from build123d import *

# Parameters (mm, degrees)
SKETCH_W            = 101
SKETCH_H            = 96
PAD_DEPTH           = 23
SKETCH001_W         = 97
SKETCH001_H         = 92
POCKET_DEPTH        = 21
SKETCH002_R         = 6
PAD001_DEPTH        = 5.6
SKETCH003_R         = 1.6
POCKET001_DEPTH     = 7
SKETCH004_R         = 1.6
POCKET002_DEPTH     = 5
SKETCH005_W         = 79
SKETCH005_H         = 52
POCKET003_DEPTH     = 23.001
SKETCH006_R         = 3
PAD002_DEPTH        = 6
POCKET004_DEPTH     = 2.001
LINEARPATTERN_COUNT = 4
LINEARPATTERN_PITCH = 3.333333
SKETCH008_R         = 4
POCKET005_DEPTH     = 2.001
POCKET006_DEPTH     = 2.001
SKETCH010_R         = 3
POCKET007_DEPTH     = 0.5
POCKET008_DEPTH     = 0.5
SKETCH012_W         = 26.5
SKETCH012_H         = 3.3
POCKET009_DEPTH     = 3
CHAMFER_SIZE        = 1.5
FILLET_R            = 1.5
CHAMFER001_SIZE     = 0.5
CHAMFER002_SIZE     = 0.49
SKETCH013_R         = 3.1
POCKET010_DEPTH     = 2.6
CHAMFER003_SIZE     = 1.3


with BuildPart() as part:
    # Sketch → Pad (new body)
    with BuildSketch(Plane.XZ):
        with Locations((50.5, 48)):
            Rectangle(SKETCH_W, SKETCH_H)
    extrude(amount=PAD_DEPTH)

    # Sketch001 (on Face5 of Pad) → Pocket (cut)
    with BuildSketch(Plane(origin=(0, 0, 0), x_dir=(1, 0, 0), z_dir=(0, 1, 0))):
        with Locations((50.5, -48)):
            Rectangle(SKETCH001_W, SKETCH001_H)
    extrude(amount=-POCKET_DEPTH, mode=Mode.SUBTRACT)

    # Sketch002 (on Face11 of Pocket) → Pad001 (join)
    with BuildSketch(Plane(origin=(0, -21, 0), x_dir=(1, 0, 0), z_dir=(0, 1, 0))):
        with Locations((94.5, -89.5)):
            Circle(SKETCH002_R)
        with Locations((94.5, -24.5)):
            Circle(SKETCH002_R)
        with Locations((6.5, -24.5)):
            Circle(SKETCH002_R)
        with Locations((6.5, -89.5)):
            Circle(SKETCH002_R)
    extrude(amount=PAD001_DEPTH)

    # Sketch003 (on Face17 of Pad001) → Pocket001 (cut)
    with BuildSketch(Plane(origin=(0, -15.4, 0), x_dir=(1, 0, 0), z_dir=(0, 1, 0))):
        with Locations((6.5, -24.5)):
            Circle(SKETCH003_R)
        with Locations((94.5, -24.5)):
            Circle(SKETCH003_R)
        with Locations((6.5, -89.5)):
            Circle(SKETCH003_R)
        with Locations((94.5, -89.5)):
            Circle(SKETCH003_R)
    extrude(amount=-POCKET001_DEPTH, mode=Mode.SUBTRACT)

    # Sketch004 (on Face14 of Pocket001) → Pocket002 (cut)
    with BuildSketch(Plane(origin=(0, -15.4, 0), x_dir=(1, 0, 0), z_dir=(0, 1, 0))):
        with Locations((6.5, -24.5)):
            Circle(SKETCH004_R)
        with Locations((94.5, -24.5)):
            Circle(SKETCH004_R)
        with Locations((94.5, -89.5)):
            Circle(SKETCH004_R)
        with Locations((6.5, -89.5)):
            Circle(SKETCH004_R)
    extrude(amount=-POCKET002_DEPTH, mode=Mode.SUBTRACT)

    # Sketch005 (on Face5 of Pocket002) → Pocket003 (cut, through all)
    with BuildSketch(Plane.XZ.offset(23)):
        with Locations((50.5, 57)):
            Rectangle(SKETCH005_W, SKETCH005_H)
    extrude(amount=-POCKET003_DEPTH, mode=Mode.SUBTRACT)

    # Sketch006 (on Face15 of Pocket003) → Pad002 (join)
    with BuildSketch(Plane(origin=(0, -21, 0), x_dir=(1, 0, 0), z_dir=(0, 1, 0))):
        with Locations((53, -13.15)):
            Circle(SKETCH006_R)
    extrude(amount=PAD002_DEPTH)

    # Sketch007 (on Face15 of Pad002) → Pocket004 (cut, through all)
    with BuildSketch(Plane(origin=(0, -21, 0), x_dir=(1, 0, 0), z_dir=(0, 1, 0))):
        with BuildLine():
            ThreePointArc((75, -8), (74.25, -7.25), (73.5, -8))
            Line((73.5, -8), (73.5, -18))
            ThreePointArc((73.5, -18), (74.25, -18.75), (75, -18))
            Line((75, -8), (75, -18))
        make_face()
    pocket004 = extrude(amount=-POCKET004_DEPTH, mode=Mode.SUBTRACT)

    # LinearPattern: Pocket004 ×4
    with Locations(*[(-i * LINEARPATTERN_PITCH, 0, 0) for i in range(1, LINEARPATTERN_COUNT)]):
        add(pocket004, mode=Mode.SUBTRACT)

    # Sketch008 (on Face31 of LinearPattern) → Pocket005 (cut, through all)
    with BuildSketch(Plane(origin=(0, -21, 0), x_dir=(1, 0, 0), z_dir=(0, 1, 0))):
        with Locations((86.85, -13.15)):
            Circle(SKETCH008_R)
    extrude(amount=-POCKET005_DEPTH, mode=Mode.SUBTRACT)

    # Sketch009 (on Face32 of Pocket005) → Pocket006 (cut, through all)
    with BuildSketch(Plane(origin=(0, -21, 0), x_dir=(1, 0, 0), z_dir=(0, 1, 0))):
        Polygon((57.701562, -14.851562), (57.701562, -11.448438), (54.701562, -8.448438), (40.701562, -8.448438), (37.701562, -11.448438), (37.701562, -23.851562), (36.901562, -23.851562), (36.901562, -11.318438), (40.571562, -7.648438), (54.836522, -7.648438), (58.501562, -11.313478), (58.501562, -14.986522), (54.836522, -18.651562), (46.101562, -18.651562), (43.501562, -21.251562), (43.501562, -23.851562), (42.701562, -23.851562), (42.701562, -20.851562), (45.701562, -17.851562), (54.701562, -17.851562), align=None)
    extrude(amount=-POCKET006_DEPTH, mode=Mode.SUBTRACT)

    # Sketch010 (on Face52 of Pocket006) → Pocket007 (cut)
    with BuildSketch(Plane(origin=(0, -21, 0), x_dir=(1, 0, 0), z_dir=(0, 1, 0))):
        Polygon((42.701561, -23.851564), (37.701561, -23.851566), (37.701561, -11.448439), (40.732891, -8.470233), (54.701561, -8.470233), (57.701562, -11.448438), (57.701562, -14.851564), (54.701561, -17.851564), (45.701561, -17.851564), (42.701561, -20.851564), align=None)
        with Locations((53, -13.15)):
            Circle(SKETCH010_R, mode=Mode.SUBTRACT)
    extrude(amount=-POCKET007_DEPTH, mode=Mode.SUBTRACT)

    # Sketch011 (on Face5 of Pocket007) → Pocket008 (cut)
    with BuildSketch(Plane.XZ.offset(23)):
        Polygon((46, 16.7), (47.5, 16.7), (49.5, 14.054249), (51.5, 16.7), (53, 16.7), (50.354249, 13.2), (53, 9.7), (51.5, 9.7), (49.5, 12.345751), (47.5, 9.7), (46, 9.7), (48.645751, 13.2), align=None)
    extrude(amount=-POCKET008_DEPTH, mode=Mode.SUBTRACT)

    # Sketch012 (on Face2 of Pocket008) → Pocket009 (cut)
    with BuildSketch(Plane(origin=(0, 0, 0), x_dir=(0, 0, -1), z_dir=(-1, 0, 0))):
        with Locations((-56.25, 6.65)):
            Rectangle(SKETCH012_W, SKETCH012_H)
    extrude(amount=-POCKET009_DEPTH, mode=Mode.SUBTRACT)

    # Chamfer
    chamfer_edges = [part.edges().sort_by_distance(p)[0] for p in [
        (0, -8.3, 56.25),
        (0, -6.65, 69.5),
        (0, -6.65, 43),
        (0, -5, 56.25),
    ]]
    chamfer(chamfer_edges, length=CHAMFER_SIZE)

    # Fillet
    fillet_edges = [part.edges().sort_by_distance(p)[0] for p in [
        (101, -11.5, 96),
        (101, -11.5, 0),
        (0, -11.5, 96),
        (0, -11.5, 0),
        (0, -23, 48),
        (50.5, -23, 0),
        (101, -23, 48),
        (50.5, -23, 96),
    ]]
    fillet(fillet_edges, radius=FILLET_R)

    # Chamfer001
    chamfer001_edges = [part.edges().sort_by_distance(p)[0] for p in [
        (44.801562, -23, 19.951562),
        (58.501562, -23, 13.15),
        (56.669042, -23, 16.819042),
        (50.469042, -23, 18.651562),
    ]]
    chamfer(chamfer001_edges, length=CHAMFER001_SIZE)

    # Chamfer002
    chamfer002_edges = [part.edges().sort_by_distance(p)[0] for p in [
        (40.201561, -21.5, 23.851565),
    ]]
    chamfer(chamfer002_edges, length=CHAMFER002_SIZE)

    # Sketch013 (on Face4 of Chamfer002) → Pocket010 (cut)
    with BuildSketch(Plane.XZ.offset(23)):
        with Locations((94.5, 89.5)):
            Circle(SKETCH013_R)
        with Locations((6.5, 89.5)):
            Circle(SKETCH013_R)
        with Locations((6.5, 24.5)):
            Circle(SKETCH013_R)
        with Locations((94.5, 24.5)):
            Circle(SKETCH013_R)
    extrude(amount=-POCKET010_DEPTH, mode=Mode.SUBTRACT)

    # Chamfer003
    chamfer003_edges = [part.edges().sort_by_distance(p)[0] for p in [
        (4.9, -20.4, 89.5),
        (4.9, -20.4, 24.5),
        (92.9, -20.4, 24.5),
        (92.9, -20.4, 89.5),
    ]]
    chamfer(chamfer003_edges, length=CHAMFER003_SIZE)


solid = part.part
Input: part model. Units: mm. Frame: model coordinates. A direction names the side the tool comes from. Round coordinates to 2 decimals unless told otherwise and drop trailing zeros. Order: outer loops, then holes, each group sorted by start corner. A loop starts at its lowest first (then second) coordinate and runs counter-clockwise, first axis right, second up.
1. Mould query, pull axis Z, two halves, no side actions, for faces 5 (the face through (50, -11, 0)), 6 (the face through (27.8, 0, 94.4)), 7 (the face through (12.497, -18.239, 24.703)), 8 (the face through (6.292, -17.224, 22.914)). Classes: released by +Z, released by -Z, zero draft, split by the parting line, or undercut.
The answers:
face 5: released by -Z
face 6: zero draft
face 7: undercut
face 8: undercut
2. Cut plane B-B, the plane z = 60. Output: boundary loops of the cut face in (x, y).
The answers:
outline: (0, -21.5) arc R1.5 ccw to (1.5, -23) - (11, -23) - (11, -21) - (2, -21) - (2, -8.3) - (1.5, -8.3) - (0, -9.8) - close; (0, -3.5) - (1.5, -5) - (2, -5) - (2, 0) - (0, 0) - close; (90, -23) - (99.5, -23) arc R1.5 ccw to (101, -21.5) - (101, 0) - (99, 0) - (99, -21) - (90, -21) - close
3. Pin query (flat end, axial travel): P1, Ø6, axis at x = 49, z = 18, coming from the +Y side; P2, Ø3, axis at x = 6.5, z = 89.5, coming from the +Y side; P3, Ø1.6, axis at y = -22.5, z = 12, coming from the +X side; P4, Ø0.8, axis at x = 50, y = -22.5, coming from the +Z side. Return the tip coordinate at first contact, or that it passes through.
The answers:
P1: stops at y = -21
P2: passes through
P3: stops at x = 100.99
P4: stops at z = 95.87
4. Cut plane A-A, the plane x = 28.5. Output: boundary loops of the cut face in (y, z).
The answers:
outline: (-23, 1.5) arc R1.5 ccw to (-21.5, 0) - (0, 0) - (0, 2) - (-21, 2) - (-21, 31) - (-23, 31) - close; (-23, 83) - (-21, 83) - (-21, 94) - (0, 94) - (0, 96) - (-21.5, 96) arc R1.5 ccw to (-23, 94.5) - close
5. Material intervals for line 1 (Z direction, x = 94.5, y = -16.7); line 2 (Z direction, x = 59.5, y = -16.5); line 3 (X direction, y = -13.75, z = 85.5), sorted ascending.
The answers:
line 1: z = 0 to 2, 18.5 to 22.9, 26.1 to 30.5, 83.5 to 87.9, 91.1 to 96
line 2: z = 0 to 2, 94 to 96
line 3: x = 0 to 2, 99 to 101
6. Cut plane D-D, the plane x = 86.85. Output: boundary loops of the cut face in (y, z).
The answers:
outline: (-23, 1.5) arc R1.5 ccw to (-21.5, 0) - (0, 0) - (0, 2) - (-21, 2) - (-21, 9.15) - (-23, 9.15) - close; (-23, 17.15) - (-21, 17.15) - (-21, 31) - (-23, 31) - close; (-23, 83) - (-21, 83) - (-21, 94) - (0, 94) - (0, 96) - (-21.5, 96) arc R1.5 ccw to (-23, 94.5) - close
7. Cut plane C-C, the plane y = -17.25. State how many separate pieces and enclosed holes the cut face has, then the cut area to 3 significant figures.
The answers:
separate pieces: 2
enclosed holes: 7
area: 1,170 mm2
8. Set-up query: faces 1 (the face through (44.82, -21.74, 19.933)), 2 (the face through (0, -11, 47)), 3 (the face through (99, -10, 49)), 4 (the face through (4.04, -21.718, 22.614)). Return all of +Z, -Z, +X, -X, +Y, -Y with unobstructed straight access to the full face (end or side cutting, diameter ignored); none if empty.
The answers:
face 1: +Y, -Y
face 2: +Z, -Z, -X, +Y, -Y
face 3: +Y
face 4: -Y
